Here's how the part is built. I have some questions about the finished solid (model axes, mm). Face numbers are marked on the shaded views. A direction names the side the tool comes from. Round coordinates to 2 decimals unless told otherwise and drop trailing zeros. Order: outer loops, then holes, each group sorted by start corner. A loop starts at its lowest first (then second) coordinate and runs counter-clockwise, first axis right, second up. Notation, with made-up numbers: (41.25, 5) - (96.25, 5) arc R24 ccw to (96.25, 16) - close; hole circle Ø6 at (35, 13.5). An arc over 180 degrees is marked (long way). Answer as a JSON object with one key per item and string values.
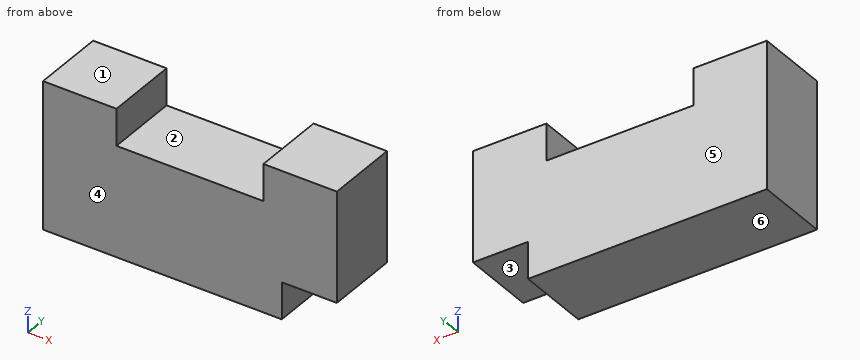
```python
from build123d import *

# Parameters (mm, degrees)
F0_W     = 101.6
F0_H     = 50.8
F1_DEPTH = 12.7
F2_W     = 19.05
F2_H     = 12.7
F3_DEPTH = 25.401
F4_W     = 50.8
F4_H     = 12.7
F5_DEPTH = 25.401


with BuildPart() as f1:
    # F0 (on Front) → F1 (new body, symmetric)
    with BuildSketch(Plane.XZ):
        Rectangle(F0_W, F0_H)
    extrude(amount=F1_DEPTH, both=True)

    # F2 (on face) → F3 (cut, through all)
    with BuildSketch(Plane.XZ.offset(12.7)):
        with Locations((41.275, -19.05)):
            Rectangle(F2_W, F2_H)
    extrude(amount=-F3_DEPTH, mode=Mode.SUBTRACT)

    # F4 (on face) → F5 (cut, through all)
    with BuildSketch(Plane.XZ.offset(12.7)):
        with Locations((0, 19.05)):
            Rectangle(F4_W, F4_H)
    extrude(amount=-F5_DEPTH, mode=Mode.SUBTRACT)


solid = f1.part
```
1. Imagine slicing it at B-B (y = -9). List the corners of the cut face in (x, z) for me, plus the area to 3 significant figures.
Responses:
{"outline": "(-50.8, -25.4) - (31.75, -25.4) - (31.75, -12.7) - (50.8, -12.7) - (50.8, 25.4) - (25.4, 25.4) - (25.4, 12.7) - (-25.4, 12.7) - (-25.4, 25.4) - (-50.8, 25.4) - close", "area": "4,270 mm2"}
2. Thinking about a two-plate mould opening in Y: for the marked faces 4, 5 and 6, which applies, pulls with the +Y half, pulls with the -Y half, needs draft (parallel to the pull), parting line crosses it, or undercut?
Responses:
{"face 4": "pulls with the -Y half", "face 5": "pulls with the +Y half", "face 6": "needs draft"}
3. For P1, Ø1.5, axis at y = 9.5, z = -18, coming from the +X side, with a flat end and sliding along its axis, tell me the tip position at first contact or that it passes through.
Responses:
{"P1": "x = 31.75"}
4. Imagine slicing it at D-D (z = -19.5). List the corners of the cut face in (x, y) for me.
Responses:
{"outline": "(-50.8, -12.7) - (31.75, -12.7) - (31.75, 12.7) - (-50.8, 12.7) - close"}
5. For the marked faces 1, 2 and 3, which set-ups out of +Z, -Z, +X, -X, +Y, -Y let a thin tool reach every point of the face, with its end or its side?
Responses:
{"face 1": "+Z, +X, -X, +Y, -Y", "face 2": "+Z, +Y, -Y", "face 3": "-Z, +X, +Y, -Y"}
6. If I drill on L1, parallel to X at y = 6.75, z = 16; L2, parallel to X at y = -5.5, z = -18; L3, parallel to Z at x = 22, y = 4.5, over which ranges is the centre line in solid material (lowest first)? Write a range as [from, to].
Responses:
{"L1": "[-50.8, -25.4], [25.4, 50.8]", "L2": "[-50.8, 31.75]", "L3": "[-25.4, 12.7]"}
7. Imagine slicing it at A-A (z = 15). List the corners of the cut face in (x, y) for me.
Responses:
{"outline": "(-50.8, -12.7) - (-25.4, -12.7) - (-25.4, 12.7) - (-50.8, 12.7) - close; (25.4, -12.7) - (50.8, -12.7) - (50.8, 12.7) - (25.4, 12.7) - close"}
8. Imagine slicing it at C-C (x = -15.5). List the corners of the cut face in (y, z) for me, plus the area to 3 significant figures.
Responses:
{"outline": "(-12.7, -25.4) - (12.7, -25.4) - (12.7, 12.7) - (-12.7, 12.7) - close", "area": "968 mm2"}
